Work out the finished part from the listing and answer in its coordinate system (mm). A direction names the side the tool comes from. Give positions to 0.01 mm unless a question says otherwise; leave off trailing zeros. Loops run counter-clockwise (first coordinate to the right, second up) from the corner with the lowest first, then second, coordinate; pieces in that order, holes last. Notation, with made-up numbers: M -21,20.25 L -17,20.25 A21 cw -17,29.25 Z; hole C 76,-9.75 d3. An arc over 180 degrees is marked long. Use a Markdown table: item, result.
```python
from build123d import *

# Parameters (mm, degrees)
SKETCH1_R           = 55
BOSS_EXTRUDE1_DEPTH = 3
CUT_EXTRUDE1_DEPTH  = 78.839578622
SKETCH4_R           = 1.5
CUT_EXTRUDE2_DEPTH  = 78.839578622


with BuildPart() as part:
    # Sketch1 → Boss-Extrude1 (new body)
    with BuildSketch(Plane.XY):
        Circle(SKETCH1_R)
    extrude(amount=BOSS_EXTRUDE1_DEPTH)

    # Sketch3 → Cut-Extrude1 (cut, through all)
    with BuildSketch(Plane.XY.offset(3)):
        with BuildLine():
            ThreePointArc((-15.937895201, 38.477482749), (-14.36842651, 42.266515347), (-18.157459108, 43.835984038))
            ThreePointArc((-18.157459108, 43.835984038), (-33.550609665, 33.550609665), (-43.835984038, 18.157459108))
            ThreePointArc((-43.835984038, 18.157459108), (-42.266515347, 14.36842651), (-38.477482749, 15.937895201))
            ThreePointArc((-38.477482749, 15.937895201), (-29.449390335, 29.449390335), (-15.937895201, 38.477482749))
        make_face()
        with BuildLine():
            ThreePointArc((18.157459108, 43.835984038), (14.36842651, 42.266515347), (15.937895201, 38.477482749))
            ThreePointArc((15.937895201, 38.477482749), (29.449390335, 29.449390335), (38.477482749, 15.937895201))
            ThreePointArc((38.477482749, 15.937895201), (42.266515347, 14.36842651), (43.835984038, 18.157459108))
            ThreePointArc((43.835984038, 18.157459108), (33.550609665, 33.550609665), (18.157459108, 43.835984038))
        make_face()
        with BuildLine():
            ThreePointArc((43.835984038, -18.157459108), (42.266515347, -14.36842651), (38.477482749, -15.937895201))
            ThreePointArc((38.477482749, -15.937895201), (29.449390335, -29.449390335), (15.937895201, -38.477482749))
            ThreePointArc((15.937895201, -38.477482749), (14.36842651, -42.266515347), (18.157459108, -43.835984038))
            ThreePointArc((18.157459108, -43.835984038), (33.550609665, -33.550609665), (43.835984038, -18.157459108))
        make_face()
        with BuildLine():
            ThreePointArc((-18.157459108, -43.835984038), (-14.36842651, -42.266515347), (-15.937895201, -38.477482749))
            ThreePointArc((-15.937895201, -38.477482749), (-29.449390335, -29.449390335), (-38.477482749, -15.937895201))
            ThreePointArc((-38.477482749, -15.937895201), (-42.266515347, -14.36842651), (-43.835984038, -18.157459108))
            ThreePointArc((-43.835984038, -18.157459108), (-33.550609665, -33.550609665), (-18.157459108, -43.835984038))
        make_face()
    extrude(amount=-CUT_EXTRUDE1_DEPTH, mode=Mode.SUBTRACT)

    # Sketch4 → Cut-Extrude2 (cut, through all)
    with BuildSketch(Plane.XY.offset(3)):
        with Locations((-17, 17)):
            Circle(SKETCH4_R)
        with Locations((17, 17)):
            Circle(SKETCH4_R)
        with Locations((17, -17)):
            Circle(SKETCH4_R)
        with Locations((-17, -17)):
            Circle(SKETCH4_R)
        Polygon((-12.5, 12.5), (-27.5, 12.5), (-27.5, -12.5), (-12.5, -12.5), (12.5, -12.5), (12.5, 12.5), align=None)
    extrude(amount=-CUT_EXTRUDE2_DEPTH, mode=Mode.SUBTRACT)


solid = part.part
```
(1) Which of the six approach directions +Z, -Z, +X, -X, +Y, -Y give full straight-line access (tool end or side, diameter ignored) to faces 1 (the cylindrical face through (33.4, -33.7, 1.5)), 2 (the flat face through (-1, 13, 0))?
Entries:
| item | result |
|---|---|
| face 1 | +Z, -Z |
| face 2 | -Z, +X, -X, +Y, -Y |
(2) A cutting plane is placed at B-B (x = 0). Write down the section's boundary in (y, z).
Entries:
| item | result |
|---|---|
| outline | M -55,0 L -12.5,0 L -12.5,3 L -55,3 Z; M 12.5,0 L 55,0 L 55,3 L 12.5,3 Z |
(3) The mould has two halves that part along Y. Classify faces 3 (the cylindrical face through (15.89, 18.01, 1.52)), 4 (the flat face through (-1, 13, 3)): released by +Y, released by -Y, zero draft, split by the parting line, or undercut.
Entries:
| item | result |
|---|---|
| face 3 | undercut |
| face 4 | zero draft |
(4) A cutting plane is placed at A-A (y = 0). Write down the section's boundary in (x, z), and give its area (3 significant figures).
Entries:
| item | result |
|---|---|
| outline | M -55,0 L -27.5,0 L -27.5,3 L -55,3 Z; M 12.5,0 L 55,0 L 55,3 L 12.5,3 Z |
| area | 210 mm² |
(5) Given P1, Ø1.5, axis at x = -38.5, z = 0.5, coming from the +Y side; P2, Ø1.5, axis at x = -6, z = 1, coming from the +Y side; P3, Ø0.9, axis at y = -5.5, z = 2, coming from the +X side; P4, Ø2.5, axis at x = -17, y = 17, coming from the -Z side, each flat-ended and moving along its own axis, determine where each tip first touches the part or whether it passes through.
Entries:
| item | result |
|---|---|
| P1 | stops at y = 40 |
| P2 | stops at y = 54.75 |
| P3 | stops at x = 54.77 |
| P4 | passes through |
(6) Consider probe 1 along Y at (x, z) = (36.5, 1.75); probe 2 along Y at (x, z) = (-17, 1.9); probe 3 along X at (y, z) = (20, 0.4). Determine where each line is inside the solid, lowest interval first. Write a range as [from, to].
Entries:
| item | result |
|---|---|
| probe 1 | y = [-41.14, -30.32], [-20.06, 20.06], [30.32, 41.14] |
| probe 2 | y = [-52.31, -44.06], [-38.02, -18.5], [-15.5, -12.5], [12.5, 15.5], [18.5, 38.02], [44.06, 52.31] |
| probe 3 | x = [-51.23, -43.03], [-36.53, 36.53], [43.03, 51.23] |
(7) A cutting plane is placed at C-C (z = 1.2). Count the separate pieces of the cut face and the enclosed holes in it, and give its area (3 significant figures).
Entries:
| item | result |
|---|---|
| separate pieces | 1 |
| enclosed holes | 9 |
| area | 7,560 mm² |
(8) A cutting plane is placed at D-D (x = 35). Write down the section's boundary in (y, z), and give its area (3 significant figures).
Entries:
| item | result |
|---|---|
| outline | M -42.43,0 L -32.04,0 L -32.04,3 L -42.43,3 Z; M -22.57,0 L 22.57,0 L 22.57,3 L -22.57,3 Z; M 32.04,0 L 42.43,0 L 42.43,3 L 32.04,3 Z |
| area | 198 mm² |
